Source: CAD feature listing. Evaluate the final solid. Frame: model axes, mm. A direction names the side the tool comes from. Round coordinates to 2 decimals unless told otherwise and drop trailing zeros. Order: outer loops, then holes, each group sorted by start corner. A loop starts at its lowest first (then second) coordinate and runs counter-clockwise, first axis right, second up. Notation, with made-up numbers: M 88,-29 L 131,-29 A17 cw 131,0 Z; hole C -18,11.5 d10. An arc over 180 degrees is marked long. Use CSV: the item, a comma, the result in double quotes. Start each with the question number.
```python
from build123d import *

# Parameters (mm, degrees)
SKETCH1_W                      = 101.6
SKETCH1_H                      = 101.6
BOSS_EXTRUDE1_DEPTH            = 3.175
F_6_32_TAPPED_HOLE1_AT_2_COUNT = 2
F_6_32_TAPPED_HOLE1_AT_2_PITCH = 88.9
SKETCH8_R                      = 1.905
CUT_EXTRUDE2_DEPTH             = 3.175


with BuildPart() as part:
    # Sketch1 → Boss-Extrude1 (new body)
    with BuildSketch(Plane.XY):
        with Locations((50.8, 50.8)):
            Rectangle(SKETCH1_W, SKETCH1_H)
    extrude(amount=BOSS_EXTRUDE1_DEPTH)

    # Sketch7 → 6-32 Tapped Hole1 (revolve, cut)
    with BuildSketch(Plane(origin=(95.25, 101.6, 1.5875), x_dir=(0, 0, 1), z_dir=(1, 0, 0))):
        Polygon((0, 0), (0, 15.79869403), (1.35255, 14.986), (1.35255, 0), align=None)
    f_6_32_tapped_hole1 = revolve(axis=Axis((95.25, 107.95, 1.5875), (0, -1, 0)), mode=Mode.SUBTRACT)

    # 6-32 Tapped Hole1 at 2: 6-32 Tapped Hole1 ×2
    with Locations(*[(-i * F_6_32_TAPPED_HOLE1_AT_2_PITCH, 0, 0) for i in range(1, F_6_32_TAPPED_HOLE1_AT_2_COUNT)]):
        add(f_6_32_tapped_hole1, mode=Mode.SUBTRACT)

    # Mirror1: 6-32 Tapped Hole1 across plane
    add(f_6_32_tapped_hole1.mirror(Plane(origin=(0, 50.8, 0), x_dir=(0, 0, 1), z_dir=(0, -1, 0))), mode=Mode.SUBTRACT)

    # Mirror1 copy 1 sketch → Mirror1 copy 1 (revolve, cut)
    with BuildSketch(Plane(origin=(6.35, 0, 1.5875), x_dir=(0, 0, 1), z_dir=(1, 0, 0))):
        Polygon((0, 0), (0, -15.79869403), (1.35255, -14.986), (1.35255, 0), align=None)
    revolve(axis=Axis((6.35, -6.35, 1.5875), (0, -1, 0)), mode=Mode.SUBTRACT)

    # Sketch8 → Cut-Extrude2 (cut)
    with BuildSketch(Plane.XY):
        with Locations(Location((19.05, 65.2145, 0), (0, 0, 180))):
            Circle(SKETCH8_R)
        with Locations(Location((19.05, 4.7625, 0), (0, 0, 180))):
            Circle(SKETCH8_R)
        with Locations(Location((82.55, 4.7625, 0), (0, 0, 180))):
            Circle(SKETCH8_R)
        with Locations(Location((82.55, 65.2145, 0), (0, 0, 180))):
            Circle(SKETCH8_R)
    extrude(amount=CUT_EXTRUDE2_DEPTH, mode=Mode.SUBTRACT)


solid = part.part
```
(1) Line query: line 1 along Y through (x, z) = (19.05, 1); line 2 along Z through (x, y) = (95, 3) (3 decimals); line 3 along X through (y, z) = (93.5, 2.6). Output: solid intervals per line, ascending.
(2) Reachability of faces 1 (the face through (0, 50, 2)), 2 (the face through (93.91, 94.21, 1.41)), 3 (the face through (93.91, 7.39, 1.41)) from +Z, -Z, +X, -X, +Y, -Y: full face, straight path, thin tool, end or side. Return the list, or none.
(3) Section B-B on z = 2.1. Give the number of separate pieces and of enclosed holes in the cut face, plus the area to 3 significant figures.
(4) Contact query for flat-ended pins moving along their axis: P1, Ø5, axis at x = 82.55, y = 4.76, coming from the -Z side; P2, Ø3, axis at x = 82.55, y = 65.21, coming from the +Z side. Output: stop coordinate, or through.
(5) Section A-A on x = 19.05. Return loops of the section in (y, z) (1 decimal).
(6) Draft query along Y for faces 4 (the face through (17.29, 5.49, 1.57)), 5 (the face through (6.15, 15.66, 1.71)), 6 (the face through (101.6, 50, 2)). Return one class per face: pulls with the +Y half, pulls with the -Y half, needs draft (parallel to the pull), parting line crosses it, or undercut.
Results below:
1,line 1,"y = 0 to 2.86, 6.67 to 63.31, 67.12 to 101.6"
1,line 2,"z = 0 to 0.258, 2.917 to 3.175"
1,line 3,"x = 0 to 5.45, 7.25 to 94.35, 96.15 to 101.6"
2,face 1,"+Z, -Z, -X, +Y, -Y"
2,face 2,"+Y"
2,face 3,"-Y"
3,separate pieces,"1"
3,enclosed holes,"4"
3,area,"10,100 mm2"
4,P1,"stops at z = 0"
4,P2,"passes through"
5,outline,"M 0,0 L 2.9,0 L 2.9,3.2 L 0,3.2 Z; M 6.7,0 L 63.3,0 L 63.3,3.2 L 6.7,3.2 Z; M 67.1,0 L 101.6,0 L 101.6,3.2 L 67.1,3.2 Z"
6,face 4,"undercut"
6,face 5,"pulls with the -Y half"
6,face 6,"needs draft"
